For this review, take the finished solid that the model builds, in its own axes (mm). Coordinates: 2 decimals unless noted, no trailing zeros. Loops run counter-clockwise (first coordinate to the right, second up) from the corner with the lowest first, then second, coordinate; pieces in that order, holes last. Notation, with made-up numbers: (21.5, -39.75) - (41.5, -39.75) arc R20 ccw to (41.5, -35.75) - close; hole circle Ø1 at (-17, 71). An arc over 180 degrees is marked (long way). Answer as a JSON object with one key per item and string values. Group by question number.
Item 1: We need section C-C (z = 4.25). Give the boundary of the cut face in (x, y), then the cut area to 3 significant figures.
Item 2: We need section A-A (y = 6.4). Give the boundary of the cut face in (x, z).
Item 3: Mouldability with a two-part tool opening along X and no side actions: class faces 1 (the cylindrical face through (-6.94, 3.93, 4.93)), 2 (the flat face through (-10.779, 5, 5)), 3 (the flat face through (0, 5, 0)), 4 (the cylindrical face through (9.216, 5.835, 4.93)) as released by +X, released by -X, zero draft, split by the parting line, or undercut.
Item 4: To check wall thickness, follow line 1 (X direction, y = 5.5, z = 0.75); line 2 (X direction, y = 3.9, z = 1.75); line 3 (Y direction, x = 9, z = 9). State the ranges of each line that lie inside material, in increasing order.
Item 5: We need section D-D (y = 4.9). Give the boundary of the cut face in (x, z), then the cut area to 3 significant figures.
Item 6: We need section B-B (x = -6.75). Give the boundary of the cut face in (y, z).
Autodesk Inventor part; units mm, degrees
ref_plane "YZ Plane" through (0, 0, 0) normal (1, 0, 0) x (0, 1, 0)
ref_plane "XZ Plane" through (0, 0, 0) normal (0, 1, 0) x (-1, 0, 0)
ref_plane "XY Plane" through (0, 0, 0) normal (0, 0, 1) x (1, 0, 0)
sketch "Skizze1" plane through (0, 0, 0) normal (0, 0, 1) x (1, 0, 0)
  circle A0 centre (7.7787, 5.2388) radius 1.5558
  circle A1 centre (-7.7788, 5.2387) radius 1.5558
  line L0 (10.5537, 7.874) -> (10.5537, -7.874)
  line L1 (-10.5537, -7.874) -> (-10.5537, 7.874)
  line L2 (-10.5537, 7.874) -> (10.5537, 7.874)
  line L3 (10.5537, -7.874) -> (-10.5537, -7.874)
  line L4 (-10.7788, 8.2387) -> (10.7787, 8.2387)
  line L5 (10.7787, 8.2387) -> (10.7787, 2.2388)
  line L6 (10.7787, 2.2388) -> (-10.7788, 2.2388)
  line L7 (-10.7788, 2.2388) -> (-10.7788, 8.2387)
  point P0 (0, 0)
  dimension "d2" = 3
  dimension "d3" = 3
  dimension "d4" = 3
  dimension "d5" = 3
extrude "Extrusion1" add sketch "Skizze1" along normal blind 10 contours L2 L1 L6 L7 L4 L5 L0 | L0 L6 L1 L2
properties part number "Abstandhalter_MPU"
Check sheet entries:
{
 "1": {"outline": "(-10.78, 2.24) - (10.78, 2.24) - (10.78, 8.24) - (-10.78, 8.24) - close; hole circle Ø3.11 at (-7.78, 5.24); hole circle Ø3.11 at (7.78, 5.24)", "area": "114 mm2"},
 "2": {"outline": "(-10.78, 0) - (-8.81, 0) - (-8.81, 10) - (-10.78, 10) - close; (-6.74, 0) - (6.74, 0) - (6.74, 10) - (-6.74, 10) - close; (8.81, 0) - (10.78, 0) - (10.78, 10) - (8.81, 10) - close"},
 "3": {"face 1": "undercut", "face 2": "released by -X", "face 3": "zero draft", "face 4": "undercut"},
 "4": {"line 1": "x = -10.78 to -9.31, -6.25 to 6.24, 9.31 to 10.78", "line 2": "x = -10.78 to -8.57, -6.99 to 6.99, 8.57 to 10.78", "line 3": "y = 2.24 to 4.27, 6.2 to 8.24"},
 "5": {"outline": "(-10.78, 0) - (-9.3, 0) - (-9.3, 10) - (-10.78, 10) - close; (-6.26, 0) - (6.26, 0) - (6.26, 10) - (-6.26, 10) - close; (9.3, 0) - (10.78, 0) - (10.78, 10) - (9.3, 10) - close", "area": "155 mm2"},
 "6": {"outline": "(2.24, 0) - (4.07, 0) - (4.07, 10) - (2.24, 10) - close; (6.41, 0) - (8.24, 0) - (8.24, 10) - (6.41, 10) - close"}
}
